from build123d import *

# Parameters (mm, degrees)
SKETCH1_W           = 100
SKETCH1_H           = 50
SKETCH1_W_2         = 41
SKETCH1_H_2         = 31
BOSS_EXTRUDE1_DEPTH = 10
SKETCH2_W           = 10
SKETCH2_H           = 38
BOSS_EXTRUDE2_DEPTH = 50
SKETCH10_W          = 100
SKETCH10_H          = 50
SKETCH10_R          = 2
BOSS_EXTRUDE6_DEPTH = 5
SKETCH12_W          = 1.8
SKETCH12_H          = 10
FILLET4_R           = 2
SKETCH13_W          = 100
SKETCH13_H          = 50
SKETCH13_R          = 6
BOSS_EXTRUDE7_DEPTH = 10
FILLET5_R           = 5


with BuildPart() as part:
    # Sketch1 → Boss-Extrude1 (new body)
    with BuildSketch(Plane(origin=(0, 0, 0), x_dir=(1, 0, 0), z_dir=(0, 1, 0))):
        with Locations((20, 0)):
            Rectangle(SKETCH1_W, SKETCH1_H)
        with Locations((39.5, -1.5)):
            Rectangle(SKETCH1_W_2, SKETCH1_H_2, mode=Mode.SUBTRACT)
    extrude(amount=BOSS_EXTRUDE1_DEPTH)

    # Sketch2 → Boss-Extrude2 (add)
    with BuildSketch(Plane.XY.offset(25)):
        with Locations((65, 29)):
            Rectangle(SKETCH2_W, SKETCH2_H)
    extrude(amount=-BOSS_EXTRUDE2_DEPTH)

    # Sketch10 → Boss-Extrude6 (add)
    with BuildSketch(Plane.XZ):
        with Locations((20, 0)):
            Rectangle(SKETCH10_W, SKETCH10_H)
        with Locations(Location((30, 0, 0), (0, 0, 270))):
            Circle(SKETCH10_R, mode=Mode.SUBTRACT)
    extrude(amount=BOSS_EXTRUDE6_DEPTH)

    # Sketch12 → Revolve3 (revolve)
    with BuildSketch(Plane.XY, mode=Mode.PRIVATE) as revolve3_sk:
        with Locations((32.9, -10)):
            Rectangle(SKETCH12_W, SKETCH12_H)
    revolve(revolve3_sk.sketch.rotate(Axis((30, -5, 0), (0, -1, 0)), 90), axis=Axis((30, -5, 0), (0, -1, 0)))

    # Fillet4
    fillet4_edges = [part.edges().sort_by_distance(p)[0] for p in [
        (30, -5, -3.8),
    ]]
    fillet(fillet4_edges, radius=FILLET4_R)

    # Sketch13 → Boss-Extrude7 (add)
    with BuildSketch(Plane.XZ.offset(5)):
        with Locations((20, 0)):
            Rectangle(SKETCH13_W, SKETCH13_H)
        with Locations(Location((30, 0, 0), (0, 0, 270))):
            Circle(SKETCH13_R, mode=Mode.SUBTRACT)
    extrude(amount=BOSS_EXTRUDE7_DEPTH)

    # Fillet5
    fillet5_edges = [part.edges().sort_by_distance(p)[0] for p in [
        (30, 0, 2),
    ]]
    fillet(fillet5_edges, radius=FILLET5_R - 0.0001)  # a hair under: the kernel refuses the full size


solid = part.part
Read the model definition and answer for the solid it produces. Units are mm, in the model's axes. A direction names the side the tool comes from. Give positions to 0.01 mm unless a question says otherwise; leave off trailing zeros. Write each loop counter-clockwise with the first axis right and the second up, starting at its lowest first coordinate (ties: lowest second). Pieces come first, ordered by that corner, then holes. Notation, with made-up numbers: (-9, -32) - (-4, -32) arc R23 cw to (-4, -15) - close; hole circle Ø2 at (2.5, -5). An arc over 180 degrees is marked (long way). Use CSV: the item, a comma, the result in double quotes. Start each with the question number.
Item 1: The part is cut by section C-C, the plane z = 0. Give the vertices of the cut face in (x, y), and give its area (3 significant figures).
Item 2: The part is cut by section B-B, the plane x = 30. Give the vertices of the cut face in (y, z).
Item 3: The mould has two halves that part along Z. Classify faces 5 (the flat face through (65, 48, 0)), 6 (the flat face through (39, 5, -14)), 7 (the flat face through (19, 3, 25)), 8 (the flat face through (60, 24, 0)): pulls with the +Z half, pulls with the -Z half, needs draft (parallel to the pull), parting line crosses it, or undercut.
Item 4: Consider line 1 (X direction, y = -9, z = 0); line 2 (X direction, y = -6, z = 0); line 3 (X direction, y = 7, z = 0.5). Determine where each line is inside the solid, lowest interval first.
Item 5: The part is cut by section A-A, the plane y = 5.5. Give the vertices of the cut face in (x, z).
Item 6: The part is cut by section D-D, the plane z = -20.5. Give the vertices of the cut face in (x, y), and give its area (3 significant figures).
Item 7: Flat-ended cylindrical pins translate along their axes: P1, Ø25, axis at x = 2, z = -7.5, coming from the +Y side; P2, Ø8, axis at y = 38.5, z = -9.5, coming from the -X side. Find the tip coordinate at first contact, or state that the pin passes through.
Item 8: For faces 1 (the flat face through (4, 10, 0)), 2 (the cylindrical face through (24.143, -9.93, 1.301)), 3 (the flat face through (19, 3, -25)), 4 (the flat face through (19, 5, 2)), determine the directions among +Z, -Z, +X, -X, +Y, -Y from which every point of the face is accessible in a straight line to the end or side of a thin tool.
Taken from the geometry:
1,outline,"(-30, -15) - (24, -15) - (24, -5) - (24.2, -5) arc R2 cw to (26.2, -7) - (26.2, -15) - (28, -15) - (28, -5) arc R5 ccw to (23, 0) - (19, 0) - (19, 10) - (-30, 10) - close; (32, -15) - (33.8, -15) - (33.8, -7) arc R2 cw to (35.8, -5) - (36, -5) - (36, -15) - (70, -15) - (70, 48) - (60, 48) - (60, 0) - (37, 0) arc R5 ccw to (32, -5) - close"
1,area,"2,360 mm2"
2,outline,"(-15, -25) - (10, -25) - (10, -14) - (0, -14) - (0, -7) arc R5 ccw to (-5, -2) - (-15, -2) - (-15, -3.8) - (-7, -3.8) arc R2 cw to (-5, -5.8) - (-5, -6) - (-15, -6) - close; (-15, 2) - (-5, 2) arc R5 ccw to (0, 7) - (0, 17) - (10, 17) - (10, 25) - (-15, 25) - (-15, 6) - (-5, 6) - (-5, 5.8) arc R2 cw to (-7, 3.8) - (-15, 3.8) - close"
3,face 5,"needs draft"
3,face 6,"undercut"
3,face 7,"pulls with the +Z half"
3,face 8,"undercut"
4,line 1,"-30 to 24, 26.2 to 28, 32 to 33.8, 36 to 70"
4,line 2,"-30 to 24, 25.93 to 28, 32 to 34.07, 36 to 70"
4,line 3,"-30 to 19, 60 to 70"
5,outline,"(-30, -25) - (70, -25) - (70, 25) - (-30, 25) - close; hole (19, -14) - (60, -14) - (60, 17) - (19, 17) - close"
6,outline,"(-30, -15) - (70, -15) - (70, 48) - (60, 48) - (60, 10) - (-30, 10) - close"
6,area,"2,880 mm2"
7,P1,"y = 10"
7,P2,"x = 60"
8,face 1,"+Z, -Z, -X, +Y"
8,face 2,"-Y"
8,face 3,"-Z, +X, -X, +Y, -Y"
8,face 4,"+Y"
